Part model, mm, in its own coordinate system. A direction names the side the tool comes from. Give positions to 0.01 mm unless a question says otherwise; leave off trailing zeros. Order: outer loops, then holes, each group sorted by start corner. A loop starts at its lowest first (then second) coordinate and runs counter-clockwise, first axis right, second up. Notation, with made-up numbers: (24, 4.5) - (53, 4.5) arc R11 cw to (53, 18.5) - close; hole circle Ø4 at (56.5, 11.5). An arc over 180 degrees is marked (long way). One line per item, written item: value.
```python
from build123d import *

# Parameters (mm, degrees)
PAD003_DEPTH         = 5
PAD_DEPTH            = 3.25
POCKET012_DEPTH      = 54.7
FILLET_R             = 1.5
PAD001_DEPTH         = 53.3
PAD002_DEPTH         = 53.3
POCKET_DEPTH         = 17.8
POCKET001_DEPTH      = 5
POCKET005_DEPTH      = 19.401
POCKET005_DEPTH_BACK = -2.101
POCKET011_DEPTH      = 4
FILLET001_R          = 1
FILLET002_R          = 1


with BuildPart() as body:
    # Sketch025 → Pad003 (new body, symmetric)
    with BuildSketch(Plane.XZ):
        with BuildLine():
            Line((-64.25, 2.1), (-62.062493, 4.706969))
            ThreePointArc((-60.147382, 5.6), (-61.203928, 5.365769), (-62.062493, 4.706969))
            Line((-60.147382, 5.6), (-53.45, 5.6))
            Line((-53.45, 5.6), (-53.45, 4.6))
            Line((-53.45, 4.6), (-53.7, 4.6))
            Line((-54.7, 4.6), (-53.7, 4.6))
            Line((-54.7, 4.6), (-60.263959, 4.6))
            ThreePointArc((-60.263959, 4.6), (-60.792232, 4.482885), (-61.221515, 4.153485))
            Line((-61.221515, 4.153485), (-62.944593, 2.1))
            Line((-64.25, 2.1), (-62.944593, 2.1))
        make_face()
    extrude(amount=PAD003_DEPTH, both=True)

    # Sketch028 → Pad (join, symmetric)
    with BuildSketch(Plane.XZ):
        with BuildLine():
            Line((-53.7, 3.1), (-53.7, -6.209252))
            ThreePointArc((-53.7, -6.209252), (-53.653109, -6.384252), (-53.525, -6.512361))
            Line((-53.2, -6.7), (-53.525, -6.512361))
            Line((-53.2, -7.7), (-53.2, -6.7))
            ThreePointArc((-54.7, -6.103128), (-54.26619, -7.198573), (-53.2, -7.7))
            Line((-54.7, 3.1), (-54.7, -6.103128))
            Line((-54.7, 3.1), (-54.7, 4.6))
            Line((-54.7, 4.6), (-53.7, 4.6))
            Line((-53.7, 3.1), (-53.7, 4.6))
        make_face()
    extrude(amount=PAD_DEPTH, both=True)

    # Sketch027 → Pocket012 (cut)
    with BuildSketch(Plane.YZ):
        Polygon((3.25, -3.7), (0.940599, -7.7), (3.25, -7.7), align=None)
    pocket012 = extrude(amount=-POCKET012_DEPTH, mode=Mode.SUBTRACT)

    # Mirrored001: Pocket012 across Sketch027 V_Axis
    add(pocket012.mirror(Plane(origin=(0, 0, 0), x_dir=(1, 0, 0), z_dir=(0, 1, 0))), mode=Mode.SUBTRACT)

    # Fillet
    fillet_edges = [body.edges().sort_by_distance(p)[0] for p in [
        (-53.45, -5, 5.1),
        (-53.45, 5, 5.1),
    ]]
    fillet(fillet_edges, radius=FILLET_R)


with BuildPart() as obj1:
    # Sketch001 → Pad001 (new body, symmetric)
    with BuildSketch(Plane.XZ):
        Polygon((64.25, 0), (55.9, 0), (55.9, -19.4), (-55.3, -19.4), (-55.3, 0), (-64.25, 0), (-64.25, 2.1), (-53.3, 2.1), (-53.3, -16.9), (0, -16.9), (53.3, -16.9), (53.3, 2.1), (64.25, 2.1), align=None)
    extrude(amount=PAD001_DEPTH, both=True)

    # Sketch002 → Pad002 (join, symmetric)
    with BuildSketch(Plane.XZ):
        with BuildLine():
            ThreePointArc((52.9, 2.1), (52.15, 1.35), (52.9, 0.6))
            Line((53.3, 0.6), (52.9, 0.6))
            Line((53.3, 2.1), (53.3, 0.6))
            Line((53.3, 2.1), (52.9, 2.1))
        make_face()
    pad002 = extrude(amount=PAD002_DEPTH, both=True)

    # Sketch003 → Pocket (cut)
    with BuildSketch(Plane.XY):
        with BuildLine():
            ThreePointArc((28.8, 39.3), (40.3, 27.8), (51.8, 39.3))
            Line((51.8, 39.3), (51.8, 48.3))
            ThreePointArc((51.8, 48.3), (51.214214, 49.714214), (49.8, 50.3))
            Line((30.8, 50.3), (49.8, 50.3))
            ThreePointArc((30.8, 50.3), (29.385786, 49.714214), (28.8, 48.3))
            Line((28.8, 39.3), (28.8, 48.3))
        make_face()
        with BuildLine():
            ThreePointArc((51.8, -39.3), (40.3, -27.8), (28.8, -39.3))
            Line((28.8, -39.3), (28.8, -48.3))
            ThreePointArc((28.8, -48.3), (29.385786, -49.714214), (30.8, -50.3))
            Line((30.8, -50.3), (49.8, -50.3))
            ThreePointArc((49.8, -50.3), (51.214214, -49.714214), (51.8, -48.3))
            Line((51.8, -39.3), (51.8, -48.3))
        make_face()
    pocket = extrude(amount=-POCKET_DEPTH, mode=Mode.SUBTRACT)

    # Sketch004 → Pocket001 (cut)
    with BuildSketch(Plane.XY):
        with BuildLine():
            ThreePointArc((59.35, -45.8), (59.603187, -46.603007), (60.271172, -47.11557))
            Line((60.271172, -47.11557), (64.25, -48.563745))
            Line((64.25, -42.886255), (64.25, -48.563745))
            Line((60.271172, -44.33443), (64.25, -42.886255))
            ThreePointArc((60.271172, -44.33443), (59.603187, -44.846993), (59.35, -45.65))
            Line((59.35, -45.65), (59.35, -45.8))
        make_face()
        with BuildLine():
            ThreePointArc((60.471172, 47.11557), (59.803187, 46.603007), (59.55, 45.8))
            Line((59.55, 45.8), (59.55, 45.65))
            ThreePointArc((59.55, 45.65), (59.803187, 44.846993), (60.471172, 44.33443))
            Line((60.471172, 44.33443), (64.25, 42.959049))
            Line((64.25, 48.490951), (64.25, 42.959049))
            Line((60.471172, 47.11557), (64.25, 48.490951))
        make_face()
    pocket001 = extrude(amount=POCKET001_DEPTH, mode=Mode.SUBTRACT)

    # Mirrored: Pad002, Pocket, Pocket001 across Sketch002 V_Axis
    add(pad002.mirror(Plane(origin=(0, 0, 0), x_dir=(0, -1, 0), z_dir=(1, 0, 0))))
    add(pocket.mirror(Plane(origin=(0, 0, 0), x_dir=(0, -1, 0), z_dir=(1, 0, 0))), mode=Mode.SUBTRACT)
    add(pocket001.mirror(Plane(origin=(0, 0, 0), x_dir=(0, -1, 0), z_dir=(1, 0, 0))), mode=Mode.SUBTRACT)

    # Sketch011 → Pocket005 (cut, two sides)
    with BuildSketch(Plane.XY) as pocket005_sk:
        Polygon((47.3, 7.5), (47.3, -7.5), (53.3, -7.5), (55.3, -6.5), (55.3, 6.5), (53.3, 7.5), align=None)
    extrude(amount=-POCKET005_DEPTH, mode=Mode.SUBTRACT)
    extrude(pocket005_sk.sketch, amount=-POCKET005_DEPTH_BACK, mode=Mode.SUBTRACT)

    # Sketch024 → Pocket011 (cut, symmetric)
    with BuildSketch(Plane.XZ):
        with BuildLine():
            Line((-54.9, 3), (-54.9, -6.248633))
            ThreePointArc((-54.9, -6.248633), (-54.463, -7.367173), (-53.383476, -7.893225))
            Line((-53.383476, -7.893225), (-53.3, -7.9))
            Line((-51.9, 3), (-53.3, -7.9))
            Line((-54.9, 3), (-51.9, 3))
        make_face()
    extrude(amount=POCKET011_DEPTH, both=True, mode=Mode.SUBTRACT)

    # Boolean: union Body
    add(body.part)

    # Fillet001
    fillet001_edges = [obj1.edges().sort_by_distance(p)[0] for p in [
        (-64.25, -53.3, 1.05),
        (64.25, -53.3, 1.05),
        (64.25, 53.3, 1.05),
        (-64.25, 53.3, 1.05),
    ]]
    fillet(fillet001_edges, radius=FILLET001_R)

    # Fillet002
    fillet002_edges = [obj1.edges().sort_by_distance(p)[0] for p in [
        (55.3, 6.5, -8.65),
        (55.3, -6.5, -8.65),
        (47.3, 7.5, -18.15),
        (47.3, -7.5, -18.15),
    ]]
    fillet(fillet002_edges, radius=FILLET002_R)


solid = obj1.part
```
1) Drop flat-ended pins along their axis: P1, Ø1, axis at x = 5.5, y = -41.5, coming from the +Z side; P2, Ø2.5, axis at x = 58, y = -1, coming from the -Z side; P3, Ø3, axis at x = -60, z = 4, coming from the -Y side; P4, Ø2, axis at x = -53, z = -2, coming from the -Y side. Give the stop position or say it passes through.
Answer:
P1: stops at z = -16.9
P2: stops at z = 0
P3: stops at y = -5
P4: stops at y = -53.3
2) Slice it at D-D on y = -41.5. Write the cut outline in (x, z).
Answer:
outline: (-64.25, 0) - (-55.3, 0) - (-55.3, -19.4) - (55.9, -19.4) - (55.9, 0) - (64.25, 0) - (64.25, 2.1) - (52.9, 2.1) arc R0.75 ccw to (52.9, 0.6) - (53.3, 0.6) - (53.3, -16.9) - (51.8, -16.9) - (51.8, -17.8) - (28.8, -17.8) - (28.8, -16.9) - (-28.8, -16.9) - (-28.8, -17.8) - (-51.8, -17.8) - (-51.8, -16.9) - (-53.3, -16.9) - (-53.3, 0.6) - (-52.9, 0.6) arc R0.75 ccw to (-52.9, 2.1) - (-64.25, 2.1) - close
3) Wall check: line 1 along X through (y, z) = (-22, -14.25); line 2 along X through (y, z) = (-2, -3); line 3 along Z through (x, y) = (-35.5, -3.5). Give the ranges that are in metal, low to high. Write a range as [from, to].
Answer:
line 1: x = [-55.3, -53.3], [53.3, 55.9]
line 2: x = [-55.3, -54.9], [-54.7, -53.7], [55.3, 55.9]
line 3: z = [-19.4, -16.9]
4) Two-plate mould, pull along Y, no slides. Class faces 4 (the face through (0.3, 53.3, -17.4)), 5 (the face through (60, -1, 0)), 6 (the face through (-54, -4, -3)): pulls with the +Y half, pulls with the -Y half, needs draft (parallel to the pull), parting line crosses it, or undercut.
Answer:
face 4: pulls with the +Y half
face 5: needs draft
face 6: undercut
5) Slice it at A-A on z = -14.75. Write the cut outline in (x, y).
Answer:
outline: (-55.3, -53.3) - (-53.3, -53.3) - (-53.3, 53.3) - (-55.3, 53.3) - close; (53.3, -53.3) - (55.9, -53.3) - (55.9, 53.3) - (53.3, 53.3) - (53.3, 7.5) - (54.75, 6.78) arc R1 cw to (55.3, 5.88) - (55.3, -5.88) arc R1 cw to (54.75, -6.78) - (53.3, -7.5) - close
6) Slice it at C-C on y = -17. Write the cut outline in (x, z), then the cut area to 3 significant figures.
Answer:
outline: (-64.25, 0) - (-55.3, 0) - (-55.3, -19.4) - (55.9, -19.4) - (55.9, 0) - (64.25, 0) - (64.25, 2.1) - (52.9, 2.1) arc R0.75 ccw to (52.9, 0.6) - (53.3, 0.6) - (53.3, -16.9) - (-53.3, -16.9) - (-53.3, 0.6) - (-52.9, 0.6) arc R0.75 ccw to (-52.9, 2.1) - (-64.25, 2.1) - close
area: 405 mm2
7) Slice it at B-B on x = 40.3. Write the cut outline in (y, z), then the cut area to 3 significant figures.
Answer:
outline: (-53.3, -19.4) - (53.3, -19.4) - (53.3, -16.9) - (50.3, -16.9) - (50.3, -17.8) - (27.8, -17.8) - (27.8, -16.9) - (-27.8, -16.9) - (-27.8, -17.8) - (-50.3, -17.8) - (-50.3, -16.9) - (-53.3, -16.9) - close
area: 226 mm2
8) Which spindle directions (+Z, -Z, +X, -X, +Y, -Y) get a long thin tool onto all of the face, cutting with end or side? Do faces 1 (the face through (-53.3, -1, -10)), 2 (the face through (-40, -39, -17.8)), 3 (the face through (-60, -1, 0)). Say none if no direction does.
Answer:
face 1: +Y, -Y
face 2: +Z
face 3: -Z, -X, +Y, -Y
